Could you check a few things on this model? Use its own coordinates, in mm. Face numbers are marked on the shaded views. A direction names the side the tool comes from. Give positions to 0.01 mm unless a question says otherwise; leave off trailing zeros. Loops run counter-clockwise (first coordinate to the right, second up) from the corner with the lowest first, then second, coordinate; pieces in that order, holes last. Notation, with made-up numbers: (33, -6) -> (51, -6) arc R21 ccw to (51, 26) -> close; hole circle Ø6 at (55, -25.75). An arc over 180 degrees is marked (long way). Put each result on its own line as item: value.
```python
from build123d import *

# Parameters (mm, degrees)
F0_R           = 14
F1_DEPTH       = 1
F2_R           = 12.25
F3_DEPTH       = 20
F5_R           = 10.75
F6_DEPTH       = 25
F10_R          = 1.25
F11_DEPTH      = 14.001
F11_DEPTH_BACK = 25
F12_R          = 1.25
F13_DEPTH      = 25
F13_DEPTH_BACK = 25
F14_R          = 1.25
F15_DEPTH      = 25
F15_DEPTH_BACK = 25
F16_DEPTH      = 10
F18_ANGLE      = 15
F19_COUNT      = 3


with BuildPart() as f1:
    # F0 (on Top) → F1 (new body)
    with BuildSketch(Plane.XY):
        Circle(F0_R)
    extrude(amount=F1_DEPTH)


with BuildPart() as f3:
    # F2 (on Top) → F3 (new body)
    with BuildSketch(Plane.XY):
        Circle(F2_R)
    extrude(amount=F3_DEPTH)

    # F5 (on offset) → F6 (cut)
    with BuildSketch(Plane.XY.offset(1)):
        Circle(F5_R)
    extrude(amount=F6_DEPTH, mode=Mode.SUBTRACT)

    # F10 (on Front) → F11 (cut, two sides)
    with BuildSketch(Plane.XZ) as f11_sk:
        with Locations((0, 8)):
            Circle(F10_R)
    extrude(amount=-F11_DEPTH, mode=Mode.SUBTRACT)
    extrude(f11_sk.sketch, amount=F11_DEPTH_BACK, mode=Mode.SUBTRACT)

    # F12 (on line) → F13 (cut, two sides)
    with BuildSketch(Plane(origin=(0, 0, 0), x_dir=(-0.5, -0.8660254038, 0), z_dir=(-0.8660254038, 0.5, 0))) as f13_sk:
        with Locations((0, 12)):
            Circle(F12_R)
    extrude(amount=-F13_DEPTH, mode=Mode.SUBTRACT)
    extrude(f13_sk.sketch, amount=F13_DEPTH_BACK, mode=Mode.SUBTRACT)

    # F14 (on line) → F15 (cut, two sides)
    with BuildSketch(Plane(origin=(0, 0, 0), x_dir=(0.5, -0.8660254038, 0), z_dir=(-0.8660254038, -0.5, 0))) as f15_sk:
        with Locations((0, 16)):
            Circle(F14_R)
    extrude(amount=-F15_DEPTH, mode=Mode.SUBTRACT)
    extrude(f15_sk.sketch, amount=F15_DEPTH_BACK, mode=Mode.SUBTRACT)


with BuildPart() as f16_tool:
    # F5 (on offset) → F16 (new body)
    with BuildSketch(Plane.XY.offset(1)):
        Circle(F5_R)
    extrude(amount=-F16_DEPTH)


with BuildPart() as f1_1:
    add(f1.part)

    # F16: cut by f16_tool
    add(f16_tool.part, mode=Mode.SUBTRACT)



with BuildPart() as f3_1:
    add(f3.part)

    # F16: cut by f16_tool
    add(f16_tool.part, mode=Mode.SUBTRACT)


with BuildPart() as f18:
    # F17 (on Front) → F18 (revolve)
    with BuildSketch(Plane.XZ):
        Polygon((-12.75, 2.5), (-12.25, 1), (-12.25, 5), align=None)
    revolve(axis=Axis((0, 0, 28.278902173), (0, 0, 1)), revolution_arc=F18_ANGLE)


with BuildPart() as f1_2:
    add(f1_1.part)

    add(f3_1.part)  # F19 merges F3

    add(f18.part)  # F19 merges F18
    # F19: F18 ×3 about axis
    f19_axis = Axis((0, 0, 28.278902173), (0, 0, 1))
    for i in range(1, F19_COUNT):
        add(f18.part.rotate(f19_axis, i * 360 / F19_COUNT))


solid = f1_2.part
```
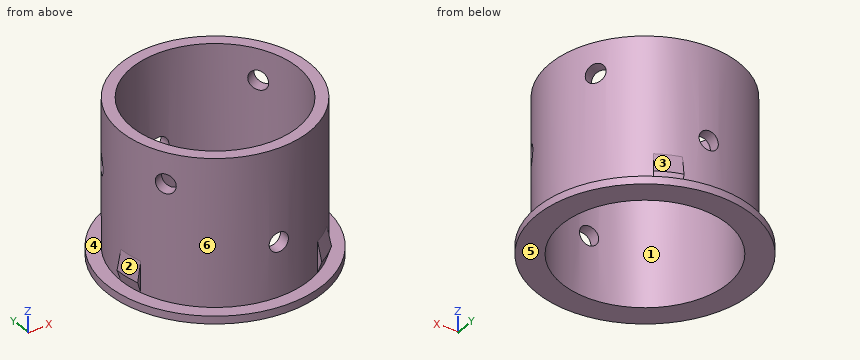
1. If we section it at A-A (x = 0): List the corners of the cut face in (y, z) for me.
Recorded:
outline: (-14, 0) -> (-10.75, 0) -> (-10.75, 6.75) -> (-12.25, 6.75) -> (-12.25, 1) -> (-14, 1) -> close; (-12.25, 9.25) -> (-10.75, 9.25) -> (-10.75, 20) -> (-12.25, 20) -> close; (10.75, 0) -> (14, 0) -> (14, 1) -> (12.25, 1) -> (12.25, 6.75) -> (10.75, 6.75) -> close; (10.75, 9.25) -> (12.25, 9.25) -> (12.25, 20) -> (10.75, 20) -> close
2. Thinking about a two-plate mould opening in X: for the marked faces 1, 2, 3 and 4, which applies, pulls with the +X half, pulls with the -X half, needs draft (parallel to the pull), parting line crosses it, or undercut?
Recorded:
face 1: undercut
face 2: pulls with the -X half
face 3: pulls with the +X half
face 4: needs draft
3. If we section it at C-C (y = 7.75): List the corners of the cut face in (x, z) for me.
Recorded:
outline: (-11.66, 0) -> (-7.45, 0) -> (-7.45, 20) -> (-9.49, 20) -> (-9.49, 1) -> (-11.66, 1) -> close; (7.45, 0) -> (11.66, 0) -> (11.66, 1) -> (9.49, 1) -> (9.49, 20) -> (7.45, 20) -> close
4. For the marked faces 5 and 6, which set-ups out of +Z, -Z, +X, -X, +Y, -Y let a thin tool reach every point of the face, with its end or its side?
Recorded:
face 5: -Z, +X, -X, +Y, -Y
face 6: +Z
5. I'm going to push flat-ended pins straight in: pin 1 (6 mm diameter, centred on x = -10.5, z = 16, fed in from -Y); pin 2 (3 mm diameter, centred on x = 0, z = 8, fed in from +Y); pin 3 (1.5 mm diameter, centred on y = -1.5, z = 14.5, fed in from -X). Where does each tip first touch, or does it pass through?
Recorded:
pin 1: stops at y = -9.69
pin 2: stops at y = 12.25
pin 3: stops at x = -12.23
6. I need wall thicknesses on line 1 (Z direction, x = 0, y = -11.15); line 2 (Y direction, x = 0, z = 10). Which ranges of each line are inside material? Lowest first, please.
Recorded:
line 1: z = 0 to 6.75, 9.25 to 20
line 2: y = -12.25 to -10.75, 10.75 to 12.25
7. If we section it at D-D (x = -5.75): List the corners of the cut face in (y, z) for me, then the cut area to 3 significant figures.
Recorded:
outline: (-12.76, 0) -> (-9.08, 0) -> (-9.08, 20) -> (-10.82, 20) -> (-10.82, 1) -> (-12.76, 1) -> close; (9.08, 0) -> (12.76, 0) -> (12.76, 1) -> (10.82, 1) -> (10.82, 20) -> (9.08, 20) -> close
area: 73.2 mm^2
